Design review of the part built by this model. Coordinates are the model's own, in mm. Round coordinates to 2 decimals unless told otherwise and drop trailing zeros. Order: outer loops, then holes, each group sorted by start corner. A loop starts at its lowest first (then second) coordinate and runs counter-clockwise, first axis right, second up. Notation, with made-up numbers: (60.25, -6.75) - (67.25, -6.75) arc R20 cw to (67.25, 14.25) - close; hole circle Ø3 at (49.25, 1.5). An arc over 180 degrees is marked (long way). Use CSV: the item, a comma, the result in double quotes.
from build123d import *

# Parameters (mm, degrees)
F0_W           = 302
F0_H           = 38
F0_W_2         = 8
F0_H_2         = 16
F1_DEPTH       = 2.5
F2_D           = 2.5
F2_CSINK_D     = 5.4
F2_CSINK_ANGLE = 90
F3_D           = 4.5
F3_CSINK_D     = 8
F3_CSINK_ANGLE = 90
F4_DEPTH       = 2.501


with BuildPart() as f1:
    # F0 (on Top) → F1 (new body)
    with BuildSketch(Plane.XY):
        Rectangle(F0_W, F0_H)
        with Locations((-136, 0)):
            Rectangle(F0_W_2, F0_H_2, mode=Mode.SUBTRACT)
        with Locations((-120, 0)):
            Rectangle(F0_W_2, F0_H_2, mode=Mode.SUBTRACT)
        with Locations((-104, 0)):
            Rectangle(F0_W_2, F0_H_2, mode=Mode.SUBTRACT)
        with Locations((-88, 0)):
            Rectangle(F0_W_2, F0_H_2, mode=Mode.SUBTRACT)
        with Locations((-72, 0)):
            Rectangle(F0_W_2, F0_H_2, mode=Mode.SUBTRACT)
        with Locations((-56, 0)):
            Rectangle(F0_W_2, F0_H_2, mode=Mode.SUBTRACT)
        with Locations((-40, 0)):
            Rectangle(F0_W_2, F0_H_2, mode=Mode.SUBTRACT)
        with Locations((-24, 0)):
            Rectangle(F0_W_2, F0_H_2, mode=Mode.SUBTRACT)
        with Locations((-8, 0)):
            Rectangle(F0_W_2, F0_H_2, mode=Mode.SUBTRACT)
        with Locations((8, 0)):
            Rectangle(F0_W_2, F0_H_2, mode=Mode.SUBTRACT)
        with Locations((24, 0)):
            Rectangle(F0_W_2, F0_H_2, mode=Mode.SUBTRACT)
        with Locations((40, 0)):
            Rectangle(F0_W_2, F0_H_2, mode=Mode.SUBTRACT)
        with Locations((56, 0)):
            Rectangle(F0_W_2, F0_H_2, mode=Mode.SUBTRACT)
        with Locations((72, 0)):
            Rectangle(F0_W_2, F0_H_2, mode=Mode.SUBTRACT)
        with Locations((88, 0)):
            Rectangle(F0_W_2, F0_H_2, mode=Mode.SUBTRACT)
        with Locations((104, 0)):
            Rectangle(F0_W_2, F0_H_2, mode=Mode.SUBTRACT)
        with Locations((120, 0)):
            Rectangle(F0_W_2, F0_H_2, mode=Mode.SUBTRACT)
        with Locations((136, 0)):
            Rectangle(F0_W_2, F0_H_2, mode=Mode.SUBTRACT)
    extrude(amount=-F1_DEPTH)

    # F2 (through all)
    with Locations(Plane.XY):
        with Locations((-128, 0), (-96, 0), (-64, 0), (-32, 0), (0, 0), (32, 0), (64, 0), (96, 0), (128, 0)):
            CounterSinkHole(F2_D / 2, F2_CSINK_D / 2, counter_sink_angle=F2_CSINK_ANGLE)

    # F3 (through all)
    with Locations(Plane.XY):
        with Locations((-146, 14), (-146, -14), (146, 14), (146, -14)):
            CounterSinkHole(F3_D / 2, F3_CSINK_D / 2, counter_sink_angle=F3_CSINK_ANGLE)

    # F0 (on Top) → F4 (cut, through all)
    with BuildSketch(Plane.XY):
        with Locations((-136, 0)):
            Rectangle(F0_W_2, F0_H_2)
    extrude(amount=-F4_DEPTH, mode=Mode.SUBTRACT)


solid = f1.part
1) To check wall thickness, follow L1, parallel to X at y = 14, z = -1.85; L2, parallel to Y at x = -146, z = -2.2; L3, parallel to Y at x = -117.5, z = -1.1. State the ranges of each line that lie inside material, in increasing order. Write a range as from..to.
Data:
L1,"x = -151..-148.25, -143.75..143.75, 148.25..151"
L2,"y = -19..-16.25, -11.75..11.75, 16.25..19"
L3,"y = -19..-8, 8..19"
2) We need section B-B (y = -5.5). Give the number of separate pieces and of enclosed holes in the cut face, then the cut area to 3 significant figures.
Data:
separate pieces,"19"
enclosed holes,"0"
area,"395 mm2"
3) We need section A-A (x = 8). Give the boundary of the cut face in (y, z).
Data:
outline,"(-19, -2.5) - (-8, -2.5) - (-8, 0) - (-19, 0) - close; (8, -2.5) - (19, -2.5) - (19, 0) - (8, 0) - close"
4) Insertion check: pin 1 Ø2 at (x, y) = (-64, 0) entering from -Z; pin 2 Ø2 at (x, y) = (-17.5, 3) entering from +Z. Each pin has a flat end and moves straight along its axis. Give the tip position at first contact, or say it passes through.
Data:
pin 1,"passes through"
pin 2,"stops at z = 0"
